Answer from the drawing. Dimensions are ordinates in mm from the lowest x, y and z of the part. A direction names the side the tool comes from. Give positions to 0.01 mm unless a question says otherwise; leave off trailing zeros. Order: outer loops, then holes, each group sorted by start corner. A loop starts at its lowest first (then second) coordinate and runs counter-clockwise, first axis right, second up.
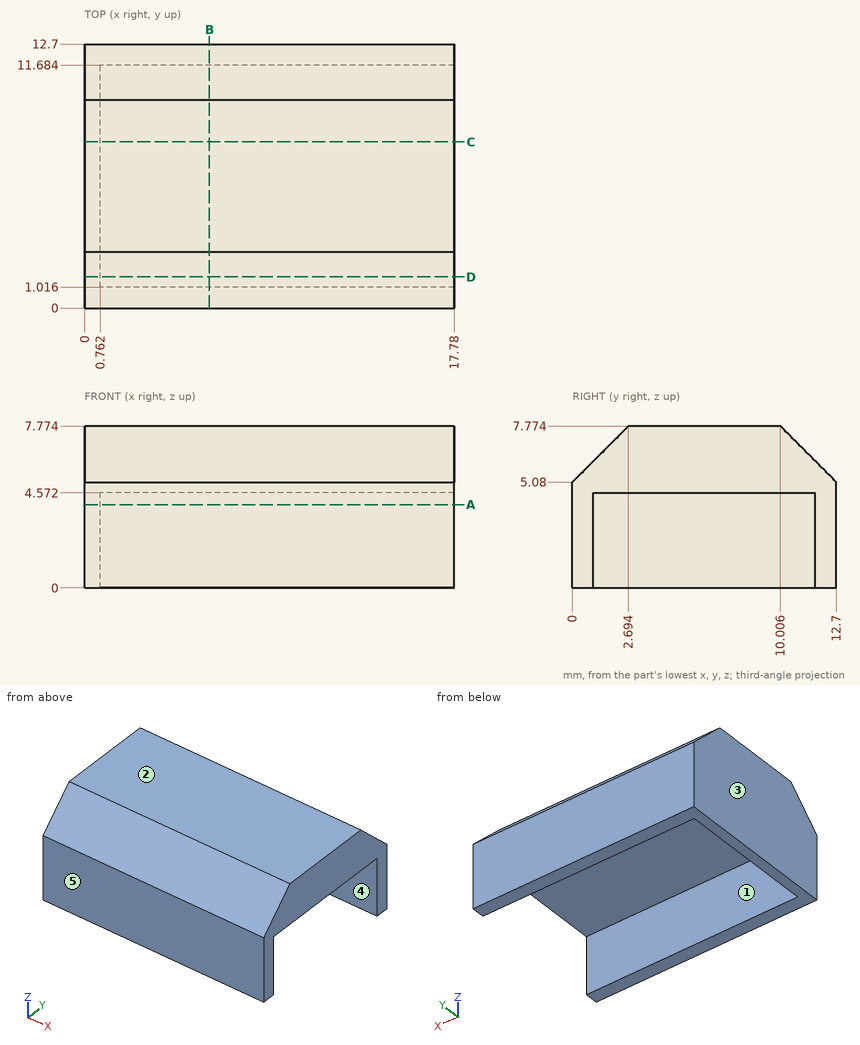
1. Straight lines are drawn through the part: probe 1 along Y at (x, z) = (8.75, 4); probe 2 along X at (y, z) = (7, 4.5); probe 3 along Z at (x, y) = (9.25, 6.25). For each, find the intervals that lie inside material, in ascending order.
Findings below:
probe 1: y = 0 to 1.02, 11.68 to 12.7
probe 2: x = 0 to 0.76
probe 3: z = 4.57 to 7.77
2. The part is cut by section A-A (z = 4). Write down the section's boundary in (x, y).
Findings below:
outline: (0, 0) - (17.78, 0) - (17.78, 1.02) - (0.76, 1.02) - (0.76, 11.68) - (17.78, 11.68) - (17.78, 12.7) - (0, 12.7) - close
3. The part is cut by section C-C (y = 8). Write down the section's boundary in (x, z).
Findings below:
outline: (0, 0) - (0.76, 0) - (0.76, 4.57) - (17.78, 4.57) - (17.78, 7.77) - (0, 7.77) - close
4. Given P1, Ø5.5, axis at x = 6, y = 8, coming from the -Z side; P2, Ø2.5, axis at y = 8, z = 2.5, coming from the +X side, each flat-ended and moving along its own axis, determine where each tip first touches the part or whether it passes through.
Findings below:
P1: stops at z = 4.57
P2: stops at x = 0.76
5. The mould has two halves that part along Y. Classify the marked faces 3, 4 and 5: pulls with the +Y half, pulls with the -Y half, needs draft (parallel to the pull), parting line crosses it, or undercut.
Findings below:
face 3: needs draft
face 4: undercut
face 5: pulls with the -Y half
6. Which of the six approach directions +Z, -Z, +X, -X, +Y, -Y give full straight-line access (tool end or side, diameter ignored) to the marked faces 1 and 2?
Findings below:
face 1: -Z, +X
face 2: +Z, +X, -X, +Y, -Y
7. The part is cut by section D-D (y = 1.5). Write down the section's boundary in (x, z), then the cut area to 3 significant figures.
Findings below:
outline: (0, 0) - (0.76, 0) - (0.76, 4.57) - (17.78, 4.57) - (17.78, 6.58) - (0, 6.58) - close
area: 39.2 mm2
8. The part is cut by section B-B (x = 6). Write down the section's boundary in (y, z), then the cut area to 3 significant figures.
Findings below:
outline: (0, 0) - (1.02, 0) - (1.02, 4.57) - (11.68, 4.57) - (11.68, 0) - (12.7, 0) - (12.7, 5.08) - (10.01, 7.77) - (2.69, 7.77) - (0, 5.08) - close
area: 42.7 mm2
